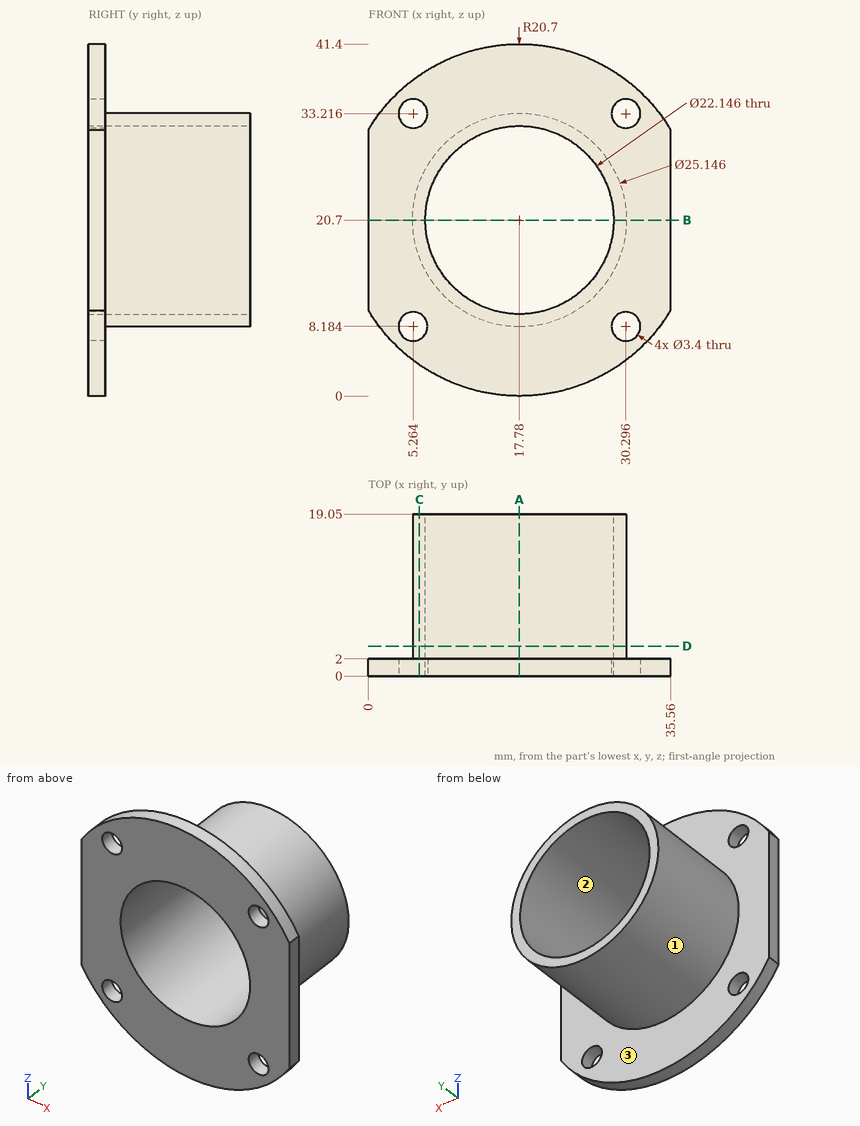
Input: dimensioned drawing with shaded views. Units: mm. Origin: part minimum x, y, z. Coordinates: 2 decimals unless noted, no trailing zeros. Order: outer loops, then holes, each group sorted by start corner. A loop starts at its lowest first (then second) coordinate and runs counter-clockwise, first axis right, second up.
1. Cut plane D-D, the plane y = 3.5. Return loops of the section in (x, z), plus the area to 3 significant figures.
Checked values:
outline: circle Ø25.15 at (17.78, 20.7); hole circle Ø22.15 at (17.78, 20.7)
area: 111 mm2
2. Contact query for flat-ended pins moving along their axis: P1, Ø13.5, axis at x = 17.78, z = 20.7, coming from the -Y side; P2, Ø2, axis at x = 4, z = 15.5, coming from the +Y side; P3, Ø8, axis at x = 8.5, y = 7, coming from the +Z side; P4, Ø8, axis at x = 14, y = 16.5, coming from the +Z side. Output: stop coordinate, or through.
Checked values:
P1: passes through
P2: stops at y = 2
P3: stops at z = 32.11
P4: stops at z = 33.27
3. Cut plane A-A, the plane x = 17.78. Return loops of the section in (y, z).
Checked values:
outline: (0, 0) - (2, 0) - (2, 8.13) - (19.05, 8.13) - (19.05, 9.63) - (0, 9.63) - close; (0, 31.77) - (19.05, 31.77) - (19.05, 33.27) - (2, 33.27) - (2, 41.4) - (0, 41.4) - close
4. Draft query along Z for the marked faces 1, 2 and 3. Return one class per face: +Z half, -Z half, draft (parallel to the pull), parting line (faces both ways), or undercut.
Checked values:
face 1: parting line
face 2: undercut
face 3: draft
5. Ray query, line 1 along Y through (x, z) = (34, 16.5); line 2 along Z through (x, y) = (23.5, 8); line 3 along X through (y, z) = (7.5, 12). Return the intervals inside material, ascending.
Checked values:
line 1: y = 0 to 2
line 2: z = 9.5 to 11.22, 30.18 to 31.9
line 3: x = 8.7 to 10.93, 24.63 to 26.86
6. Cut plane C-C, the plane x = 6. Return loops of the section in (y, z).
Checked values:
outline: (0, 3.68) - (2, 3.68) - (2, 6.65) - (0, 6.65) - close; (0, 9.72) - (2, 9.72) - (2, 16.31) - (19.05, 16.31) - (19.05, 25.09) - (2, 25.09) - (2, 31.68) - (0, 31.68) - close; (0, 34.75) - (2, 34.75) - (2, 37.72) - (0, 37.72) - close
7. Cut plane B-B, the plane z = 20.7. Return loops of the section in (x, y).
Checked values:
outline: (0, 0) - (6.71, 0) - (6.71, 19.05) - (5.21, 19.05) - (5.21, 2) - (0, 2) - close; (28.85, 0) - (35.56, 0) - (35.56, 2) - (30.35, 2) - (30.35, 19.05) - (28.85, 19.05) - close
